Can you work these out from the model? Positions are in its coordinate system, mm. A direction names the side the tool comes from. Round coordinates to 2 decimals unless told otherwise and drop trailing zeros. Loops run counter-clockwise (first coordinate to the right, second up) from the corner with the lowest first, then second, coordinate; pieces in that order, holes last. Notation, with made-up numbers: (-18.5, -0.75) -> (37.5, -0.75) arc R6 cw to (37.5, 6.25) -> close; hole circle Ø2 at (7, 13.25). An arc over 180 degrees is marked (long way). Use a Markdown table: item, result.
from build123d import *

# Parameters (mm, degrees)
F0_W        = 100
F0_H        = 55
F1_DEPTH    = 50
F2_T        = -5.5
F3_T1_DEPTH = 202.8673195186


# Not quite as in the source:
# - a fillet or chamfer that OpenCascade refuses, or shapes differently, is made with other operations: its cross-section is extruded or revolved along the edge and cut away or added


with BuildPart() as f1:
    # F0 (on Front) → F1 (new body)
    with BuildSketch(Plane.XZ):
        Rectangle(F0_W, F0_H)
    extrude(amount=F1_DEPTH)

    # F2
    f2_openings = [f1.faces().sort_by_distance(p)[0] for p in [
        (0, -25, 27.5),
    ]]
    offset(amount=F2_T, openings=f2_openings)

    # F3: chamfer of 20 on 1 edges, made by hand

    # F3_s2 → F3_t1 (cut)
    with BuildSketch(Plane.YZ.offset(-101.4336597593)):
        Polygon((0, 7.5), (-20, 27.5), (0, 27.5), align=None)
    extrude(amount=F3_T1_DEPTH, mode=Mode.SUBTRACT)


solid = f1.part
1. I want a section at A-A (z = 9.5). Please give me the cut outline in (x, y), plus the area to 3 significant figures.
Answer sheet:
| item | result |
|---|---|
| outline | (-50, -50) -> (50, -50) -> (50, -2) -> (-50, -2) -> close; hole (-44.5, -44.5) -> (44.5, -44.5) -> (44.5, -5.5) -> (-44.5, -5.5) -> close |
| area | 1,330 mm² |
2. I want a section at C-C (x = -36). Please give me the cut outline in (y, z).
Answer sheet:
| item | result |
|---|---|
| outline | (-50, -27.5) -> (0, -27.5) -> (0, 7.5) -> (-5.5, 13) -> (-5.5, -22) -> (-44.5, -22) -> (-44.5, 27.5) -> (-50, 27.5) -> close |
3. I want a section at D-D (z = -21). Please give me the cut outline in (x, y), plus the area to 3 significant figures.
Answer sheet:
| item | result |
|---|---|
| outline | (-50, -50) -> (50, -50) -> (50, 0) -> (-50, 0) -> close; hole (-44.5, -44.5) -> (44.5, -44.5) -> (44.5, -5.5) -> (-44.5, -5.5) -> close |
| area | 1,530 mm² |
4. I need wall thicknesses on line 1 (X direction, y = -34.5, z = 24); line 2 (Y direction, x = 12, z = -3.5); line 3 (Z direction, x = -20.5, y = -24.5). Which ranges of each line are inside material? Lowest first, please.
Answer sheet:
| item | result |
|---|---|
| line 1 | x = -50 to -44.5, 44.5 to 50 |
| line 2 | y = -50 to -44.5, -5.5 to 0 |
| line 3 | z = -27.5 to -22 |
5. I want a section at B-B (y = -28). Please give me the cut outline in (x, z).
Answer sheet:
| item | result |
|---|---|
| outline | (-50, -27.5) -> (50, -27.5) -> (50, 27.5) -> (44.5, 27.5) -> (44.5, -22) -> (-44.5, -22) -> (-44.5, 27.5) -> (-50, 27.5) -> close |
6. If we mould it in two halves opening along X, with no side actions, what happens to faces 1 (the flat face through (44.5, -25, 2)), 2 (the flat face through (-1, -25, -22)), 3 (the flat face through (-50, -25, 0)), 4 (the flat face through (-1, -25, -27.5))? For each: +X half, -X half, draft (parallel to the pull), parting line (faces both ways), or undercut.
Answer sheet:
| item | result |
|---|---|
| face 1 | undercut |
| face 2 | undercut |
| face 3 | -X half |
| face 4 | draft |
7. Will these pins go through, and if not, where does the flat tip stop? pin 1 Ø5 at (x, y) = (-24, -12) entering from +Z; pin 2 Ø6 at (x, z) = (-30.5, 17) entering from +Y.
Answer sheet:
| item | result |
|---|---|
| pin 1 | stops at z = -22 |
| pin 2 | stops at y = -44.5 |
8. Which directions (+Z, -Z, +X, -X, +Y, -Y) give clear straight access to the entire face, cutting with the end or side of a thin tool? Please do faces 5 (the flat face through (-8, -45, 27.5)), 6 (the flat face through (-44.5, -25, 2)).
Answer sheet:
| item | result |
|---|---|
| face 5 | +Z, +X, -X, +Y, -Y |
| face 6 | +Z |
